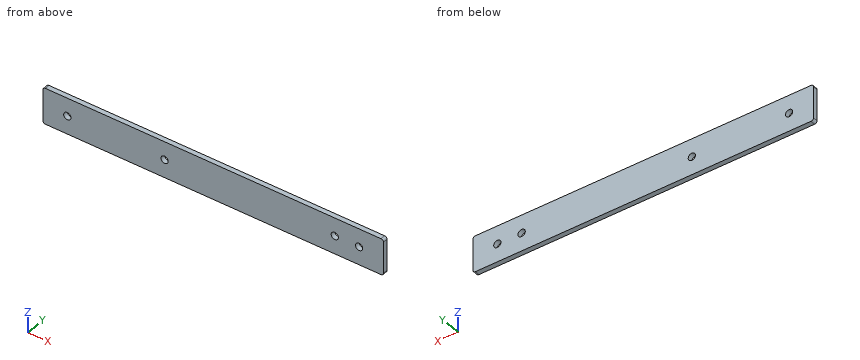
```python
from build123d import *

# Parameters (mm, degrees)
BOSS_EXTRUDE1_DEPTH = 2
FILLET1_R           = 1
SKETCH2_R           = 1.5
CUT_EXTRUDE1_DEPTH  = 10


with BuildPart() as part:
    # Sketch1 → Boss-Extrude1 (new body)
    with BuildSketch(Plane(origin=(0, 0, 0), x_dir=(1, 0, 0), z_dir=(0, 1, 0))):
        with BuildLine():
            ThreePointArc((48.5, 7.5), (50, 9), (51.5, 7.5))
            Line((51.5, 7.5), (140, 7.5))
            Line((140, 7.5), (140, 15))
            Line((140, 15), (0, 15))
            Line((0, 15), (0, 7.5))
            Line((0, 7.5), (8.5, 7.5))
            ThreePointArc((8.5, 7.5), (10, 9), (11.5, 7.5))
            Line((11.5, 7.5), (48.5, 7.5))
        make_face()
        with BuildLine():
            Line((140, 7.5), (51.5, 7.5))
            ThreePointArc((51.5, 7.5), (50, 6), (48.5, 7.5))
            Line((48.5, 7.5), (11.5, 7.5))
            ThreePointArc((11.5, 7.5), (10, 6), (8.5, 7.5))
            Line((8.5, 7.5), (0, 7.5))
            Line((0, 7.5), (0, 0))
            Line((0, 0), (140, 0))
            Line((140, 0), (140, 7.5))
        make_face()
    extrude(amount=BOSS_EXTRUDE1_DEPTH)

    # Fillet1
    fillet1_edges = [part.edges().sort_by_distance(p)[0] for p in [
        (0, 1, 0),
        (0, 1, -15),
        (140, 1, -15),
        (140, 1, 0),
    ]]
    fillet(fillet1_edges, radius=FILLET1_R)

    # Sketch2 → Cut-Extrude1 (cut)
    with BuildSketch(Plane(origin=(0, 2, 0), x_dir=(1, 0, 0), z_dir=(0, 1, 0))):
        with Locations(Location((130, 7.5, 0), (0, 0, 270))):
            Circle(SKETCH2_R)
        with Locations(Location((120, 7.5, 0), (0, 0, 270))):
            Circle(SKETCH2_R)
    extrude(amount=-CUT_EXTRUDE1_DEPTH, mode=Mode.SUBTRACT)


solid = part.part
```
Here's how the part is built. I have some questions about the finished solid (model axes, mm). Round coordinates to 2 decimals unless told otherwise and drop trailing zeros. Order: outer loops, then holes, each group sorted by start corner. A loop starts at its lowest first (then second) coordinate and runs counter-clockwise, first axis right, second up. Notation, with made-up numbers: M 24.25,64 L 58.25,64 A20 cw 58.25,76 Z; hole C 69,51 d1. An arc over 180 degrees is marked long. Answer in a Markdown table with one row per item.
Item 1: Imagine slicing it at A-A, the plane z = -7.5. Write out the boundary of the cut face in (x, y).
A:
| item | result |
|---|---|
| outline | M 0,0 L 8.5,0 L 8.5,2 L 0,2 Z; M 11.5,0 L 48.5,0 L 48.5,2 L 11.5,2 Z; M 51.5,0 L 118.5,0 L 118.5,2 L 51.5,2 Z; M 121.5,0 L 128.5,0 L 128.5,2 L 121.5,2 Z; M 131.5,0 L 140,0 L 140,2 L 131.5,2 Z |
Item 2: If I drill on L1, parallel to Z at x = 130, y = 1.3; L2, parallel to X at y = 1.15, z = -8.5; L3, parallel to Z at x = 9, y = 0.5, over which ranges is the centre line in solid material (lowest first)? Write a range as from..to.
A:
| item | result |
|---|---|
| L1 | z = -15..-9, -6..0 |
| L2 | x = 0..8.88, 11.12..48.88, 51.12..118.88, 121.12..128.88, 131.12..140 |
| L3 | z = -15..-8.62, -6.38..0 |
Item 3: Imagine slicing it at B-B, the plane x = 130. Write out the boundary of the cut face in (y, z), and give its area (3 significant figures).
A:
| item | result |
|---|---|
| outline | M 0,-15 L 2,-15 L 2,-9 L 0,-9 Z; M 0,-6 L 2,-6 L 2,0 L 0,0 Z |
| area | 24.0 mm2 |
